For this review, take the finished solid that the model builds, in its own axes (mm). A direction names the side the tool comes from. Give positions to 0.01 mm unless a question says otherwise; leave off trailing zeros. Loops run counter-clockwise (first coordinate to the right, second up) from the corner with the lowest first, then second, coordinate; pieces in that order, holes last. Notation, with made-up numbers: (3.5, -37.75) - (62.5, -37.75) arc R33 ccw to (62.5, 0.25) - close; hole circle Ø6 at (2.25, -23). An arc over 180 degrees is marked (long way). Answer in a Markdown table with one row per item.
```python
from build123d import *

# Parameters (mm, degrees)
F0_W      = 44.45
F0_H      = 31.75
F1_DEPTH  = 25.4
F2_W      = 31.75
F2_H      = 19.05
F3_DEPTH  = 25.4
F5_DEPTH  = 12.7
F7_DEPTH  = 12.7
F9_DEPTH  = 25.4
F10_R     = 6.35
F11_DEPTH = 25.4


with BuildPart() as f1:
    # F0 (on Front) → F1 (new body)
    with BuildSketch(Plane.XZ):
        with Locations((22.225, 15.875)):
            Rectangle(F0_W, F0_H)
    extrude(amount=F1_DEPTH)

    # F2 (on face) → F3 (cut)
    with BuildSketch(Plane.XZ.offset(25.4)):
        with Locations((28.575, 22.225)):
            Rectangle(F2_W, F2_H)
    extrude(amount=-F3_DEPTH, mode=Mode.SUBTRACT)

    # F4 (on face) → F5 (join)
    with BuildSketch(Plane.XY.offset(12.7)):
        with BuildLine():
            Line((44.45, 0), (44.45, -25.4))
            ThreePointArc((44.45, -25.4), (57.15, -12.7), (44.45, 0))
        make_face()
    extrude(amount=-F5_DEPTH)

    # F6 (on face) → F7 (join)
    with BuildSketch(Plane.YZ.offset(12.7)):
        with BuildLine():
            Line((-25.4, 31.75), (0, 31.75))
            ThreePointArc((0, 31.75), (-12.7, 44.45), (-25.4, 31.75))
        make_face()
    extrude(amount=-F7_DEPTH)

    # F8 (on face) → F9 (cut)
    with BuildSketch(Plane.YZ.offset(12.7)):
        with BuildLine():
            Line((-19.05, 42.7485226281), (-19.05, 31.75))
            ThreePointArc((-19.05, 31.75), (-12.7, 25.4), (-6.35, 31.75))
            Line((-6.35, 31.75), (-6.35, 42.7485226281))
            ThreePointArc((-6.35, 42.7485226281), (-12.7, 44.45), (-19.05, 42.7485226281))
        make_face()
    extrude(amount=-F9_DEPTH, mode=Mode.SUBTRACT)

    # F10 (on face) → F11 (cut)
    with BuildSketch(Plane.XY.offset(12.7)):
        with Locations((44.45, -12.7)):
            Circle(F10_R)
        with Locations((25.4, -12.7)):
            Circle(F10_R)
    extrude(amount=-F11_DEPTH, mode=Mode.SUBTRACT)


solid = f1.part
```
1. Clearance check with flat-ended pins moving along their axes: pin 1 (7.5 mm diameter, centred on x = 37.5, y = -13.5, fed in from +Z); pin 2 (12 mm diameter, centred on y = -20, z = 31.5, fed in from +X); pin 3 (3.5 mm diameter, centred on x = 8.5, z = 38.5, fed in from -Y). State where each tip first meets the part, or that it passes through.
Values:
| item | result |
|---|---|
| pin 1 | stops at z = 12.7 |
| pin 2 | stops at x = 12.7 |
| pin 3 | stops at y = -24.37 |
2. We need section A-A, the plane x = 25.4. Give the boundary of the cut face in (y, z), and give its area (3 significant figures).
Values:
| item | result |
|---|---|
| outline | (-25.4, 0) - (-19.05, 0) - (-19.05, 12.7) - (-25.4, 12.7) - close; (-6.35, 0) - (0, 0) - (0, 12.7) - (-6.35, 12.7) - close |
| area | 161 mm^2 |
3. For faces 4 (the face through (20.36, -16.56, 6.44)), 5 (the face through (35, -13, 12.7)), 6 (the face through (6, -19.05, 37)), list the 3-axis set-ups (+Z, -Z, +X, -X, +Y, -Y) from which the entire face can be reached by the end or side of a thin tool; tool diameter is ignored.
Values:
| item | result |
|---|---|
| face 4 | +Z, -Z |
| face 5 | +Z, +X, +Y, -Y |
| face 6 | +Z, +X, -X |
4. We need section C-C, the plane z = 31. Give the boundary of the cut face in (x, y).
Values:
| item | result |
|---|---|
| outline | (0, -25.4) - (12.7, -25.4) - (12.7, -19.01) - (0, -19.01) - close; (0, -6.39) - (12.7, -6.39) - (12.7, 0) - (0, 0) - close |
5. We need section D-D, the plane x = 10.5. Give the boundary of the cut face in (y, z), and give its area (3 significant figures).
Values:
| item | result |
|---|---|
| outline | (-25.4, 0) - (0, 0) - (0, 31.75) arc R12.7 ccw to (-6.35, 42.75) - (-6.35, 31.75) arc R6.35 cw to (-19.05, 31.75) - (-19.05, 42.75) arc R12.7 ccw to (-25.4, 31.75) - close |
| area | 842 mm^2 |
6. We need section B-B, the plane y = -12.7. Give the boundary of the cut face in (x, z).
Values:
| item | result |
|---|---|
| outline | (0, 0) - (19.05, 0) - (19.05, 12.7) - (12.7, 12.7) - (12.7, 25.4) - (0, 25.4) - close; (31.75, 0) - (38.1, 0) - (38.1, 12.7) - (31.75, 12.7) - close; (50.8, 0) - (57.15, 0) - (57.15, 12.7) - (50.8, 12.7) - close |
7. Mouldability with a two-part tool opening along X and no side actions: class faces 1 (the face through (12.7, -13, 25)), 2 (the face through (17, 0, 9)), 3 (the face through (50.316, -15.132, 6.439)) as released by +X, released by -X, zero draft, split by the parting line, or undercut.
Values:
| item | result |
|---|---|
| face 1 | released by +X |
| face 2 | zero draft |
| face 3 | undercut |
8. Wall thickness on line 1 (Y direction, x = 25, z = 6); line 2 (X direction, y = -18.25, z = 5.5); line 3 (X direction, y = -11.75, z = 4): over which ranges is each line inside the solid? List them lowest first. Write a range as [from, to].
Values:
| item | result |
|---|---|
| line 1 | y = [-25.4, -19.04], [-6.36, 0] |
| line 2 | x = [0, 22.31], [28.49, 41.36], [47.54, 55.87] |
| line 3 | x = [0, 19.12], [31.68, 38.17], [50.73, 57.11] |
